Read the model definition and answer for the solid it produces. Units are mm, in the model's axes. Face numbers are marked on the shaded views. A direction names the side the tool comes from. Coordinates: 2 decimals unless noted, no trailing zeros. Write each loop counter-clockwise with the first axis right and the second up, starting at its lowest first coordinate (ties: lowest second). Pieces come first, ordered by that corner, then holes. Notation, with made-up numbers: (77, -4) - (84, -4) arc R19 cw to (84, 3) - close; hole circle Ø4 at (78, 60). An arc over 180 degrees is marked (long way). Return JSON: item names as keys, results as strings.
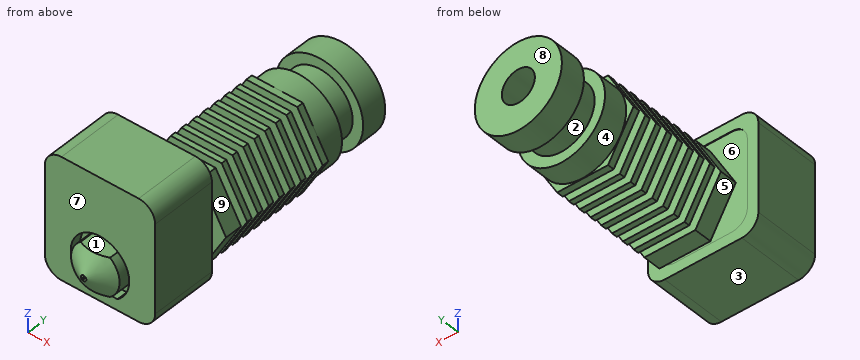
```python
from build123d import *

# Parameters (mm, degrees)
BOSS_EXTRU_1_DEPTH         = 21.8
ESQUISSE3_R                = 9.237604307
ESQUISSE3_R_2              = 4
ENL_V_MAT_EXTRU_1_DEPTH    = 1.3
R_P_TITION_LIN_AIRE1_COUNT = 8
R_P_TITION_LIN_AIRE1_PITCH = 2.3
ESQUISSE6_W                = 16
ESQUISSE6_H                = 18
BOSS_EXTRU_2_DEPTH         = 10
ESQUISSE9_W                = 8.8
ESQUISSE9_H                = 0.9
ENL_V_MAT_EXTRU_2_DEPTH    = 5.5
ESQUISSE10_R               = 3
ENL_V_MAT_EXTRU_3_DEPTH    = 42.790519287
CONG_1_R                   = 2.8
BOSS_EXTRU_3_DEPTH         = 2
BOSS_EXTRU_3_DEPTH_BACK    = 10.1
ESQUISSE13_W               = 20
ESQUISSE13_H               = 22
CONG_2_R                   = 3
BOSS_EXTRU_4_DEPTH         = 2
ESQUISSE15_R               = 3
ENL_V_MAT_EXTRU_4_DEPTH    = 7


with BuildPart() as part:
    # Esquisse1 → Révolution1 (revolve)
    with BuildSketch(Plane.XY):
        Polygon((0, 35.5), (-7.9, 35.5), (-7.9, 30.8), (-6, 30.8), (-6, 26.3), (-7.9, 26.3), (-7.9, 21.8), (-4, 21.8), (-4, 0), (0, 0), align=None)
    revolve(axis=Axis((0, 35.5, 0), (0, -1, 0)))

    # Esquisse2 → Boss.-Extru.1 (add)
    with BuildSketch(Plane.XZ):
        Polygon((-4.618802154, -8), (4.618802154, -8), (9.237604307, 0), (4.618802154, 8), (-4.618802154, 8), (-9.237604307, 0), align=None)
    extrude(amount=-BOSS_EXTRU_1_DEPTH)

    # Esquisse3 → Enlèv. mat.-Extru.1 (cut)
    with BuildSketch(Plane(origin=(0, 3.2, 0), x_dir=(-1, 0, 0), z_dir=(0, -1, 0))):
        Circle(ESQUISSE3_R)
        with Locations(Location((0, 0, 0), (0, 0, 180))):
            Circle(ESQUISSE3_R_2, mode=Mode.SUBTRACT)
    enl_v_mat_extru_1 = extrude(amount=-ENL_V_MAT_EXTRU_1_DEPTH, mode=Mode.SUBTRACT)

    # Répétition linéaire1: Enlèv. mat.-Extru.1 ×8
    with Locations(*[(0, i * R_P_TITION_LIN_AIRE1_PITCH, 0) for i in range(1, R_P_TITION_LIN_AIRE1_COUNT)]):
        add(enl_v_mat_extru_1, mode=Mode.SUBTRACT)

    # Esquisse5 → Révolution2 (revolve)
    with BuildSketch(Plane(origin=(0, 0, 0), x_dir=(0, 0, -1), z_dir=(1, 0, 0))):
        Polygon((-1.25, 0), (-1.25, -2), (-2.9, -2), (-2.9, -4), (0, -4), (0, 0), align=None)
    revolve(axis=Axis((0, 0, 0), (0, -1, 0)))

    # Esquisse6 → Boss.-Extru.2 (add)
    with BuildSketch(Plane.XZ.offset(4)):
        with Locations((0, 4.75)):
            Rectangle(ESQUISSE6_W, ESQUISSE6_H)
    extrude(amount=BOSS_EXTRU_2_DEPTH)

    # Esquisse8 → Révolution3 (revolve)
    with BuildSketch(Plane(origin=(0, 0, 0), x_dir=(0, 0, -1), z_dir=(1, 0, 0))):
        Polygon((0, -19.5), (-0.5, -19.5), (-4.4, -17), (-4.4, -14), (0, -14), align=None)
    revolve(axis=Axis((0, -14, 0), (0, -1, 0)))

    # Esquisse9 → Enlèv. mat.-Extru.2 (cut)
    with BuildSketch(Plane.XZ.offset(19.5)):
        with Locations((0, -3.95)):
            Rectangle(ESQUISSE9_W, ESQUISSE9_H)
        with Locations((0, 3.95)):
            Rectangle(ESQUISSE9_W, ESQUISSE9_H)
    extrude(amount=-ENL_V_MAT_EXTRU_2_DEPTH, mode=Mode.SUBTRACT)

    # Esquisse10 → Enlèv. mat.-Extru.3 (cut, through all)
    with BuildSketch(Plane.ZY.offset(8)):
        with Locations((7.95, -9)):
            Circle(ESQUISSE10_R)
    extrude(amount=-ENL_V_MAT_EXTRU_3_DEPTH, mode=Mode.SUBTRACT)

    # Congé1
    cong_1_edges = [part.edges().sort_by_distance(p)[0] for p in [
        (-8, -9, 13.75),
        (-8, -9, -4.25),
        (8, -9, -4.25),
        (8, -9, 13.75),
    ]]
    fillet(cong_1_edges, radius=CONG_1_R - 0.0001)  # a hair under: the kernel refuses the full size

    # Esquisse12 → Enlèvement de matière-Révolution1 (revolve, cut)
    with BuildSketch(Plane(origin=(0, 0, 0), x_dir=(0, 0, -1), z_dir=(1, 0, 0))):
        Polygon((0, 35.5), (-0.9, 35.5), (-0.9, -14), (-0.15, -14), (-0.15, -19.5), (0, -19.5), align=None)
    revolve(axis=Axis((0, 35.5, 0), (0, -1, 0)), mode=Mode.SUBTRACT)

    # Esquisse13 → Boss.-Extru.3 (add, two sides: drawn at the far end of the back side and taken through both)
    with BuildSketch(Plane.XZ.offset(14).offset(-BOSS_EXTRU_3_DEPTH_BACK)):
        with Locations((0, 4.75)):
            Rectangle(ESQUISSE13_W, ESQUISSE13_H)
        with BuildLine():
            Line((-5.2, 13.75), (5.2, 13.75))
            ThreePointArc((5.2, 13.75), (7.179898987, 12.929898987), (8, 10.95))
            Line((8, 10.95), (8, -1.45))
            ThreePointArc((8, -1.45), (7.179898987, -3.429898987), (5.2, -4.25))
            Line((5.2, -4.25), (-5.2, -4.25))
            ThreePointArc((-5.2, -4.25), (-7.179898987, -3.429898987), (-8, -1.45))
            Line((-8, -1.45), (-8, 10.95))
            ThreePointArc((-8, 10.95), (-7.179898987, 12.929898987), (-5.2, 13.75))
        make_face(mode=Mode.SUBTRACT)
    extrude(amount=BOSS_EXTRU_3_DEPTH + BOSS_EXTRU_3_DEPTH_BACK)

    # Congé2
    cong_2_edges = [part.edges().sort_by_distance(p)[0] for p in [
        (-10, -9.95, -6.25),
        (-10, -9.95, 15.75),
        (10, -9.95, 15.75),
        (10, -9.95, -6.25),
    ]]
    fillet(cong_2_edges, radius=CONG_2_R)

    # Esquisse14 → Boss.-Extru.4 (add)
    with BuildSketch(Plane.XZ.offset(14)):
        with BuildLine():
            Line((0, 5.3), (0, 13.75))
            Line((0, 13.75), (-5.2, 13.75))
            ThreePointArc((-5.2, 13.75), (-7.179898987, 12.929898987), (-8, 10.95))
            Line((-8, 10.95), (-8, -1.45))
            ThreePointArc((-8, -1.45), (-7.179898987, -3.429898987), (-5.2, -4.25))
            Line((-5.2, -4.25), (-3.166622807, -4.25))
            ThreePointArc((-3.166622807, -4.25), (-5.030656021, 1.668082732), (0, 5.3))
        make_face()
        with BuildLine():
            Line((5.2, 13.75), (0, 13.75))
            Line((0, 13.75), (0, 5.3))
            ThreePointArc((0, 5.3), (5.030656021, 1.668082732), (3.166622807, -4.25))
            Line((3.166622807, -4.25), (5.2, -4.25))
            ThreePointArc((5.2, -4.25), (7.179898987, -3.429898987), (8, -1.45))
            Line((8, -1.45), (8, 10.95))
            ThreePointArc((8, 10.95), (7.179898987, 12.929898987), (5.2, 13.75))
        make_face()
    extrude(amount=BOSS_EXTRU_4_DEPTH)

    # Esquisse15 → Enlèv. mat.-Extru.4 (cut)
    with BuildSketch(Plane(origin=(0, 35.5, 0), x_dir=(1, 0, 0), z_dir=(0, 1, 0))):
        with Locations(Location((0, 0, 0), (0, 0, 180))):
            Circle(ESQUISSE15_R)
    extrude(amount=-ENL_V_MAT_EXTRU_4_DEPTH, mode=Mode.SUBTRACT)


solid = part.part
```
(1) Flat-ended cylindrical pins translate along their axes: P1, Ø3, axis at x = -4, z = -2.5, coming from the -Y side; P2, Ø2, axis at x = -6.5, y = 5, coming from the +Z side; P3, Ø1, axis at x = 0, y = 2, coming from the +Z side; P4, Ø1.6, axis at x = 0, z = 0, coming from the -Y side. Find the tip coordinate at first contact, or state that the pin passes through.
Answer:
{"P1": "y = -17.76", "P2": "z = 6.47", "P3": "z = 8", "P4": "y = -19.5"}
(2) Which of the six approach directions +Z, -Z, +X, -X, +Y, -Y give full straight-line access (tool end or side, diameter ignored) to the marked faces 1, 2, 3, 4 and 5?
Answer:
{"face 1": "-Y", "face 2": "none", "face 3": "-Z, +X, -X, -Y", "face 4": "+Y", "face 5": "-Z, -X, +Y"}
(3) Determine the mould class of the marked faces 6, 7, 8 and 9 for opening direction Y: +Y half, -Y half, draft (parallel to the pull), parting line (faces both ways), or undercut.
Answer:
{"face 6": "undercut", "face 7": "-Y half", "face 8": "+Y half", "face 9": "draft"}
(4) A cutting plane is placed at A-A (y = -9). Determine the outline of the cut face in (x, z), and give its area (3 significant figures).
Answer:
{"outline": "(-10, -3.25) arc R3 ccw to (-7, -6.25) - (7, -6.25) arc R3 ccw to (10, -3.25) - (10, 12.75) arc R3 ccw to (7, 15.75) - (-7, 15.75) arc R3 ccw to (-10, 12.75) - close; hole (-8, 4.95) - (8, 4.95) - (8, 10.95) - (-8, 10.95) - close; hole circle Ø1.8 at (0, 0)", "area": "334 mm²"}
(5) A cutting plane is placed at B-B (y = 27.5). Determine the outline of the cut face in (x, z).
Answer:
{"outline": "circle Ø12 at (0, 0); hole circle Ø1.8 at (0, 0)"}
(6) Straight lines are drawn through the part: line 1 (Z direction, x = 0, y = -15.15); line 2 (Z direction, x = 0, y = -3.5); line 3 (Z direction, x = 0, y = 20). For each, find the intervals that lie inside material, in ascending order. Write a range as from..to.
Answer:
{"line 1": "-6.25..-4.25, -3.5..-0.15, 0.15..3.5, 5.3..15.75", "line 2": "-2.9..-0.9, 0.9..2.9", "line 3": "-4..-0.9, 0.9..4"}
